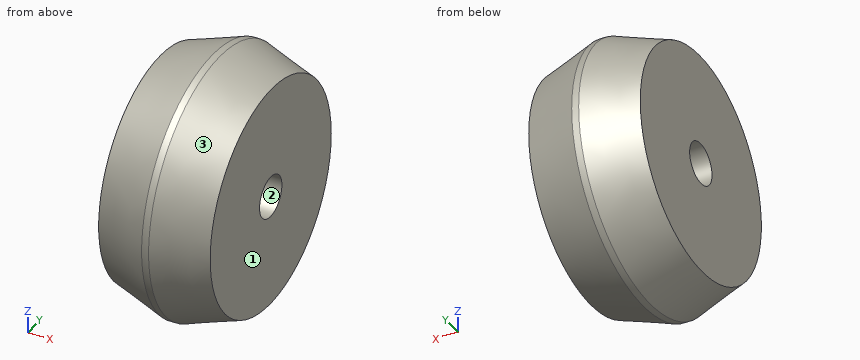
Autodesk Inventor part; units mm, degrees
ref_plane "YZ Plane" through (0, 0, 0) normal (1, 0, 0) x (0, 1, 0)
ref_plane "XZ Plane" through (0, 0, 0) normal (0, 1, 0) x (-1, 0, 0)
ref_plane "XY Plane" through (0, 0, 0) normal (0, 0, 1) x (1, 0, 0)
sketch "스케치1" plane through (0, 0, 0) normal (1, 0, 0) x (0, 1, 0)
  circle A0 centre (0, 0) radius 37.5
  dimension "d0" = 75
extrude "돌출1" add sketch "스케치1" along normal blind 32
chamfer "모따기1" distance 5 distance2 15 1 edges at (32, -37.5, 0) measured on face at (32, 9.7729, -7.7936)
chamfer "모따기2" distance 5 distance2 15 1 edges at (0, -37.5, 0) measured on face at (0, 9.7729, -7.7936)
sketch "스케치2" plane through (32, 0, 0) normal (1, 0, 0) x (0, 0, -1)
  circle A0 centre (0, 0) radius 6
  dimension "d9" = 12
extrude "돌출2" cut sketch "스케치2" against normal blind 32
properties part number "Part_Rubber" material "고무"
Could you check a few things on this model? Use its own coordinates, in mm. Face numbers are marked on the shaded views. Round coordinates to 2 decimals unless told otherwise and drop trailing zeros. Write each loop counter-clockwise with the first axis right and the second up, starting at its lowest first coordinate (ties: lowest second). Pieces come first, ordered by that corner, then holes. Notation, with made-up numbers: M 22.5,40.5 L 47.5,40.5 A22 ccw 47.5,73.5 Z; hole C 2.25,61.25 d8. An arc over 180 degrees is marked long. Answer in a Markdown table with one row per item. Add a question column.
Q1. If I drill on line 1 (Y direction, x = 25.5, z = -2); line 2 (Z direction, x = 25, y = 3); line 3 (Z direction, x = 23.5, y = -27), over which ranges is the centre line in solid material (lowest first)? Write a range as from..to.
Q2. Imagine slicing it at A-A (y = 0). Please give me the cut outline in (x, z), then the cut area to 3 significant figures.
Q3. Imagine slicing it at D-D (x = 29.5). Please give me the cut outline in (y, z).
Q4. Imagine slicing it at C-C (x = 18). Please give me the cut outline in (y, z), then the cut area to 3 significant figures.
Q5. If we mould it in two halves opening along Y, with no side actions, what happens to the marked faces 1, 2 and 3? For each: +Y half, -Y half, draft (parallel to the pull), parting line (faces both ways), or undercut.
Q6. Will these pins go through, and if not, where does the flat tip stop? pin 1 Ø2 at (y, z) = (-25, -13.5) entering from -X; pin 2 Ø8 at (x, z) = (16.5, 21) entering from -Y; pin 3 Ø9.5 at (y, z) = (0, 0) entering from +X; pin 4 Ø6 at (x, y) = (26.5, 15.5) entering from +Z.
Values:
| question | item | result |
|---|---|---|
| 1 | line 1 | -34.61..-5.66, 5.66..34.61 |
| 1 | line 2 | -34.7..-5.2, 5.2..34.7 |
| 1 | line 3 | -22.79..22.79 |
| 2 | outline | M 0,-32.5 L 15,-37.5 L 17,-37.5 L 32,-32.5 L 32,-6 L 0,-6 Z; M 0,6 L 32,6 L 32,32.5 L 17,37.5 L 15,37.5 L 0,32.5 Z |
| 2 | area | 1,870 mm^2 |
| 3 | outline | C 0,0 d66.67; hole C 0,0 d12 |
| 4 | outline | C 0,0 d74.33; hole C 0,0 d12 |
| 4 | area | 4,230 mm^2 |
| 5 | face 1 | draft |
| 5 | face 2 | undercut |
| 5 | face 3 | parting line |
| 6 | pin 1 | x = 0 |
| 6 | pin 2 | y = -33.43 |
| 6 | pin 3 | through |
| 6 | pin 4 | z = 32.39 |
